Autodesk Inventor part; units mm, degrees
ref_plane "YZ Plane" through (0, 0, 0) normal (1, 0, 0) x (0, 1, 0)
ref_plane "XZ Plane" through (0, 0, 0) normal (0, 1, 0) x (-1, 0, 0)
ref_plane "XY Plane" through (0, 0, 0) normal (0, 0, 1) x (1, 0, 0)
sketch "スケッチ1" plane through (0, 0, 0) normal (0, 0, 1) x (1, 0, 0)
  line L0 (-16, -16) -> (16, -16)
  line L1 (16, -16) -> (16, 16)
  line L2 (16, 16) -> (-16, 16)
  line L3 (-16, 16) -> (-16, -16)
  line L4 (-16, -16) -> (16, 16) construction
  line L5 (16, -16) -> (-16, 16) construction
  line L6 (-14.4, 14.4) -> (14.4, 14.4)
  line L7 (14.4, 14.4) -> (14.4, -14.4)
  line L8 (14.4, -14.4) -> (-14.4, -14.4)
  line L9 (-14.4, -14.4) -> (-14.4, 14.4)
  point P0 (0, 0)
  dimension "d0" = 32
  dimension "d1" = 32
  dimension "d2" = 1.6
extrude "押し出し1" add sketch "スケッチ1" along normal blind 110
sketch "スケッチ2" plane through (-16, 16, 0) normal (0, 1, 0) x (1, 0, 0)
  circle A0 centre (16, 0) radius 13.6
  dimension "d5" = 27.2
extrude "押し出し2" cut sketch "スケッチ2" against normal blind 32
sketch "スケッチ3" plane through (-16, 16, 110) normal (0, 1, 0) x (1, 0, 0)
  line L0 (32, 0) -> (0, 0)
  point P0 (16, 110)
  point P1 (16, 15)
  dimension "d16" = 95
hole "穴1" at (0, 16, 95) direction (0, -1, 0) diameter 10.5 end through all
sketch "スケッチ4" plane through (-16, 16, 110) normal (0, 1, 0) x (1, 0, 0)
  circle A0 centre (16, 15) radius 13.6
  point P0 (16, 110)
  dimension "d17" = 95
  dimension "d18" = 27.2
properties part number "軸受上用"
Verification items for the finished model (mm, model axes). A direction names the side the tool comes from. Coordinates: 2 decimals unless noted, no trailing zeros. Write each loop counter-clockwise with the first axis right and the second up, starting at its lowest first coordinate (ties: lowest second). Pieces come first, ordered by that corner, then holes. Notation, with made-up numbers: (25.5, 3) - (32.5, 3) arc R21 ccw to (32.5, 8) - close; hole circle Ø7 at (22.25, 72). An arc over 180 degrees is marked (long way). One line per question, with ' | ' between items. Start each with the question number.
1. Access from +Z, -Z, +X, -X, +Y, -Y to the whole of each face (thin tool, end or side, straight path). Record for faces 1 (the flat face through (0, -14.4, 54)), 2 (the cylindrical face through (-1.6, 15.2, 100)).
2. Gauge pin test, flat end, axial feed: P1, Ø8.5, axis at x = 0, z = 95, coming from the -Y side. Record the tip position at first contact, or that the pin passes through.
3. Section check B-B (x = 0). Enter the section's corners in (y, z), plus the area to 3 significant figures.
4. Section check A-A (z = 38). Enter the section's corners in (x, y), plus the area to 3 significant figures.
5. Section check C-C (z = 95). Enter the section's corners in (x, y), plus the area to 3 significant figures.
6. Section check D-D (x = 9.5). Enter the section's corners in (y, z), plus the area to 3 significant figures.
7. Draft check along X on faces 3 (the flat face through (-16, 0, 54)), 4 (the cylindrical face through (-0.299, 15.211, 13.597)), 5 (the flat face through (-15, 0, 0)). Enter one of: released by +X, released by -X, zero draft, split by the parting line, or undercut.
8. Material ranges on line 1 along X through (y, z) = (15.15, 95); line 2 along Y through (x, z) = (0, 20), recorded low to high.
Computed values:
1) face 1: +Z, -Z | face 2: +Y, -Y
2) P1: through
3) outline: (-16, 13.6) - (-14.4, 13.6) - (-14.4, 89.75) - (-16, 89.75) - close; (-16, 100.25) - (-14.4, 100.25) - (-14.4, 110) - (-16, 110) - close; (14.4, 13.6) - (16, 13.6) - (16, 89.75) - (14.4, 89.75) - close; (14.4, 100.25) - (16, 100.25) - (16, 110) - (14.4, 110) - close | area: 275 mm²
4) outline: (-16, -16) - (16, -16) - (16, 16) - (-16, 16) - close; hole (-14.4, -14.4) - (14.4, -14.4) - (14.4, 14.4) - (-14.4, 14.4) - close | area: 195 mm²
5) outline: (-16, -16) - (-5.25, -16) - (-5.25, -14.4) - (-14.4, -14.4) - (-14.4, 14.4) - (-5.25, 14.4) - (-5.25, 16) - (-16, 16) - close; (5.25, -16) - (16, -16) - (16, 16) - (5.25, 16) - (5.25, 14.4) - (14.4, 14.4) - (14.4, -14.4) - (5.25, -14.4) - close | area: 161 mm²
6) outline: (-16, 9.73) - (-14.4, 9.73) - (-14.4, 110) - (-16, 110) - close; (14.4, 9.73) - (16, 9.73) - (16, 110) - (14.4, 110) - close | area: 321 mm²
7) face 3: released by -X | face 4: undercut | face 5: zero draft
8) line 1: -16 to -5.25, 5.25 to 16 | line 2: -16 to -14.4, 14.4 to 16
